```python
from build123d import *


with BuildPart() as cone001:
    # Cone001 → Cone001 (revolve)
    with BuildSketch(Plane(origin=(0, 0, -15), x_dir=(1, 0, 0), z_dir=(0, -1, 0))):
        Polygon((0, 0), (15, 0), (4, 15), (0, 15), align=None)
    revolve(axis=Axis((0, 0, -15), (0, 0, 1)))


with BuildPart() as cone002:
    # Cone002 → Cone002 (revolve)
    with BuildSketch(Plane(origin=(0, 0, -65), x_dir=(1, 0, 0), z_dir=(0, -1, 0))):
        Polygon((0, 0), (25, 0), (15, 50), (0, 50), align=None)
    revolve(axis=Axis((0, 0, -65), (0, 0, 1)))


with BuildPart() as fusion:
    # Cone → Cone (revolve)
    with BuildSketch(Plane.XZ):
        Polygon((0, 0), (4, 0), (2, 15), (0, 15), align=None)
    revolve(axis=Axis((0, 0, 0), (0, 0, 1)))

    # Fusion: union Cone001, Cone002
    add(cone001.part)
    add(cone002.part)


solid = fusion.part
```
The model under review builds one solid part; all positions refer to its coordinate system, in mm. Coordinates: 2 decimals unless noted, no trailing zeros. Loops run counter-clockwise (first coordinate to the right, second up) from the corner with the lowest first, then second, coordinate; pieces in that order, holes last. Notation, with made-up numbers: (13.25, 72.5) -> (42.25, 72.5) arc R17 cw to (42.25, 83.5) -> close; hole circle Ø9 at (-12.5, 5). An arc over 180 degrees is marked (long way). Answer as CSV lines item,"result".
Item 1: Insertion check: pin 1 (1.5 mm diameter, centred on x = 3, z = -41, fed in from -Y); pin 2 (4 mm diameter, centred on x = 15, z = -36, fed in from +Y); pin 3 (5 mm diameter, centred on y = 8, z = -47.5, fed in from +X). Each pin has a flat end and moves straight along its axis. Give the tip position at first contact, or say it passes through.
Results below:
pin 1,"stops at y = -20.16"
pin 2,"stops at y = 14.21"
pin 3,"stops at x = 20.96"
Item 2: For L1, parallel to Y at x = -2, z = -9.5; L2, parallel to Y at x = -10, z = -27.5; L3, parallel to X at y = 7, z = -40.5, list the stretches that pass through material, from the lowest coordinate up.
Results below:
L1,"y = -10.78 to 10.78"
L2,"y = -14.36 to 14.36"
L3,"x = -18.84 to 18.84"
Item 3: Take a section at A-A, the plane y = 0. State the section outline as (x, z) points, and give its area (4 significant figures).
Results below:
outline,"(-25, -65) -> (25, -65) -> (15, -15) -> (4, 0) -> (2, 15) -> (-2, 15) -> (-4, 0) -> (-15, -15) -> close"
area,"2,375 mm2"
Item 4: Take a section at C-C, the plane z = -40.5. State the section outline as (x, y) points.
Results below:
outline,"circle Ø40.2 at (0, 0)"
Item 5: Take a section at D-D, the plane z = -52. State the section outline as (x, y) points, and give its area (3 significant figures).
Results below:
outline,"circle Ø44.8 at (0, 0)"
area,"1,580 mm2"
